```python
from build123d import *

# Parameters (mm, degrees)
SKETCH1_R           = 61.9125
BOSS_EXTRUDE1_DEPTH = 10
SKETCH4_R           = 49.9125
CUT_EXTRUDE1_DEPTH  = 5.5
CUT_EXTRUDE1_TAPER  = 30
SKETCH5_R           = 49.9125
CUT_EXTRUDE2_DEPTH  = 5.5
CUT_EXTRUDE2_TAPER  = 30
SKETCH6_R           = 17.5
BOSS_EXTRUDE2_DEPTH = 4
BOSS_EXTRUDE2_TAPER = 30
SKETCH9_R           = 17.5
BOSS_EXTRUDE3_DEPTH = 4
BOSS_EXTRUDE3_TAPER = 30
CUT_EXTRUDE4_DEPTH  = 24
SKETCH12_R          = 61.9125
SKETCH12_R_2        = 54.9125
BOSS_EXTRUDE4_DEPTH = 0.1
SKETCH14_R          = 61.9125
SKETCH14_R_2        = 54.9125
BOSS_EXTRUDE5_DEPTH = 0.1


with BuildPart() as part:
    # Sketch1 → Boss-Extrude1 (new body, symmetric)
    with BuildSketch(Plane.XY):
        Circle(SKETCH1_R)
    extrude(amount=BOSS_EXTRUDE1_DEPTH, both=True)

    # Sketch4 → Cut-Extrude1 (cut)
    with BuildSketch(Plane.XY.offset(10)):
        Circle(SKETCH4_R)
    extrude(amount=-CUT_EXTRUDE1_DEPTH, taper=CUT_EXTRUDE1_TAPER, mode=Mode.SUBTRACT)

    # Sketch5 → Cut-Extrude2 (cut)
    with BuildSketch(Plane(origin=(0, 0, -10), x_dir=(-1, 0, 0), z_dir=(0, 0, -1))):
        Circle(SKETCH5_R)
    extrude(amount=-CUT_EXTRUDE2_DEPTH, taper=CUT_EXTRUDE2_TAPER, mode=Mode.SUBTRACT)

    # Sketch6 → Boss-Extrude2 (add)
    with BuildSketch(Plane.XY.offset(4.5)):
        Circle(SKETCH6_R)
    extrude(amount=BOSS_EXTRUDE2_DEPTH, taper=BOSS_EXTRUDE2_TAPER)

    # Sketch9 → Boss-Extrude3 (add)
    with BuildSketch(Plane(origin=(0, 0, -4.5), x_dir=(-1, 0, 0), z_dir=(0, 0, -1))):
        Circle(SKETCH9_R)
    extrude(amount=BOSS_EXTRUDE3_DEPTH, taper=BOSS_EXTRUDE3_TAPER)

    # Sketch10 → Cut-Extrude4 (cut)
    with BuildSketch(Plane(origin=(0, 0, -8.5), x_dir=(-1, 0, 0), z_dir=(0, 0, -1))):
        Polygon((6.317873481, -3.014046231), (5.769177344, 3.964415817), (-0.548696137, 6.978462048), (-6.317873481, 3.014046231), (-5.769177344, -3.964415817), (0.548696137, -6.978462048), align=None)
    extrude(amount=-CUT_EXTRUDE4_DEPTH, mode=Mode.SUBTRACT)

    # Sketch12 → Boss-Extrude4 (add)
    with BuildSketch(Plane.XY.offset(10)):
        Circle(SKETCH12_R)
        Circle(SKETCH12_R_2, mode=Mode.SUBTRACT)
    extrude(amount=BOSS_EXTRUDE4_DEPTH)

    # Sketch14 → Boss-Extrude5 (add)
    with BuildSketch(Plane(origin=(0, 0, -10), x_dir=(-1, 0, 0), z_dir=(0, 0, -1))):
        Circle(SKETCH14_R)
        Circle(SKETCH14_R_2, mode=Mode.SUBTRACT)
    extrude(amount=BOSS_EXTRUDE5_DEPTH)


solid = part.part
```
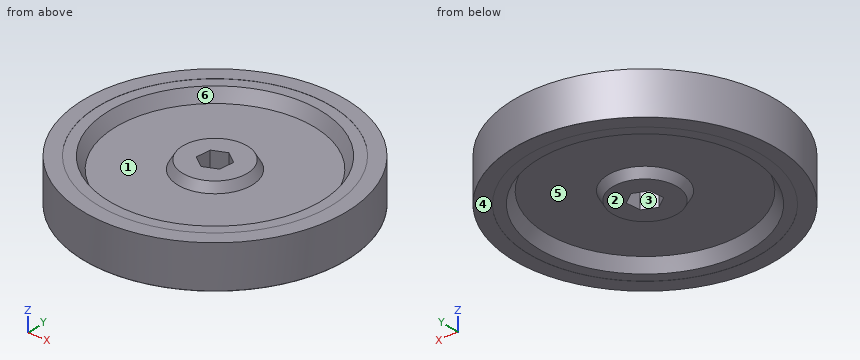
Source: CAD feature listing. Evaluate the final solid. Frame: model axes, mm. Face numbers are marked on the shaded views. A direction names the side the tool comes from. Give positions to 0.01 mm unless a question says otherwise; leave off trailing zeros. Loops run counter-clockwise (first coordinate to the right, second up) from the corner with the lowest first, then second, coordinate; pieces in that order, holes last. Notation, with made-up numbers: (74.5, 29) - (101.5, 29) arc R17 ccw to (101.5, 62) - close; hole circle Ø7 at (4.5, 55). An arc over 180 degrees is marked (long way). Use CSV: the item, a comma, the result in double quotes. Start each with the question number.
1. Ray query, L1, parallel to X at y = 2.5, z = -5.25; L2, parallel to X at y = -15, z = 5.25; L3, parallel to Y at x = -4, z = 7. Return the intervals inside material, ascending.
2. Section A-A (z = 2.75). Output: boundary loops of the cut face in (x, y) (1 decimal).
3. Draft query along X for the marked faces 4, 5 and 6. Return one class per face: +X half, -X half, draft (parallel to the pull), parting line (faces both ways), or undercut.
4. Pin query (flat end, axial travel): pin 1 (12 mm diameter, centred on x = -18, y = 8, fed in from -Z); pin 2 (1 mm diameter, centred on y = -15.5, z = 3.5, fed in from +X); pin 3 (1.5 mm diameter, centred on x = -21, y = -6.5, fed in from +Z). Return the tip coordinate at first contact, or that it passes through.
5. Reachability of the marked faces 1, 2 and 3 from +Z, -Z, +X, -X, +Y, -Y: full face, straight path, thin tool, end or side. Return the list, or none.
6. Section B-B (x = -53). Output: boundary loops of the cut face in (y, z).
Response:
1,L1,"-61.86 to -47.1, -16.88 to -5.88, 6.28 to 16.88, 47.1 to 61.86"
1,L2,"-60.07 to -44.72, -8.14 to 8.14, 44.72 to 60.07"
1,L3,"-61.78 to -48.01, -15.55 to -4.61, 4.81 to 15.55, 48.01 to 61.78"
2,outline,"circle Ø123.8 at (0, 0); hole (-6.3, -3) - (-0.5, -7) - (5.8, -4) - (6.3, 3) - (0.5, 7) - (-5.8, 4) - close"
3,face 4,"draft"
3,face 5,"undercut"
3,face 6,"undercut"
4,pin 1,"z = -8.5"
4,pin 2,"x = 60.07"
4,pin 3,"z = 4.5"
5,face 1,"+Z"
5,face 2,"-Z"
5,face 3,"+Z, -Z"
6,outline,"(-32, -10.1) - (-14.37, -10.1) - (-14.37, -10) - (14.37, -10) - (14.37, -10.1) - (32, -10.1) - (32, 10.1) - (14.37, 10.1) - (14.37, 10) - (-14.37, 10) - (-14.37, 10.1) - (-32, 10.1) - close"
